from build123d import *

# Parameters (mm, degrees)
SKETCH1_R           = 2
BOSS_EXTRUDE1_DEPTH = 5


with BuildPart() as part:
    # Sketch1 → Boss-Extrude1 (new body)
    with BuildSketch(Plane(origin=(0, 0, 0), x_dir=(1, 0, 0), z_dir=(0, 1, 0))):
        Polygon((-62.278471827, 53.688877211), (-91.278471827, 24.688877211), (-91.278471827, -88.311122789), (-62.278471827, -59.311122789), align=None)
        with Locations((-76.778471827, -17.311122789)):
            Circle(SKETCH1_R, mode=Mode.SUBTRACT)
    extrude(amount=BOSS_EXTRUDE1_DEPTH)


solid = part.part
Verification items for the finished model (mm, model axes). Coordinates: 2 decimals unless noted, no trailing zeros. Order: outer loops, then holes, each group sorted by start corner. A loop starts at its lowest first (then second) coordinate and runs counter-clockwise, first axis right, second up.
Item 1: Section check A-A, the plane y = 2.3. Enter the section's corners in (x, z), then the cut area to 3 significant figures.
Filled in:
outline: (-91.28, -24.69) - (-62.28, -53.69) - (-62.28, 59.31) - (-91.28, 88.31) - close; hole circle Ø4 at (-76.78, 17.31)
area: 3,260 mm2
Item 2: Section check B-B, the plane z = 68. Enter the section's corners in (x, y), then the cut area to 3 significant figures.
Filled in:
outline: (-91.28, 0) - (-70.97, 0) - (-70.97, 5) - (-91.28, 5) - close
area: 102 mm2
Item 3: Release check for a two-part mould opening along X. For faces 1 (the face through (-78.253, 2.465, 15.959)), 2 (the face through (-62.278, 2, 4)), 3 (the face through (-74, 5, 16)), 4 (the face through (-91.278, 2, 31)) record: +X half, -X half, draft (parallel to the pull), parting line (faces both ways), or undercut.
Filled in:
face 1: undercut
face 2: +X half
face 3: draft
face 4: -X half
Item 4: Depth check by flat-ended pin: pin 1 (3 mm diameter, centred on x = -70, y = 1.5, fed in from -Z). Enter the tip coordinate at first touch or a pass-through.
Filled in:
pin 1: stops at z = -47.47
Item 5: Section check C-C, the plane x = -73.25. Enter the section's corners in (y, z).
Filled in:
outline: (0, -42.72) - (5, -42.72) - (5, 70.28) - (0, 70.28) - close
Item 6: Material ranges on L1, parallel to Z at x = -75.75, y = 1.6; L2, parallel to Z at x = -83.25, y = 0.25; L3, parallel to X at y = 1.65, z = 63, recorded low to high.
Filled in:
L1: z = -40.22 to 15.6, 19.03 to 72.78
L2: z = -32.72 to 80.28
L3: x = -91.28 to -65.97
